Part model, mm, in its own coordinate system. Round coordinates to 2 decimals unless told otherwise and drop trailing zeros. Loops run counter-clockwise (first coordinate to the right, second up) from the corner with the lowest first, then second, coordinate; pieces in that order, holes last. Notation, with made-up numbers: (7, 18.5) - (40, 18.5) arc R29 ccw to (40, 53.5) - close; hole circle Ø8 at (47, -4). An arc over 180 degrees is marked (long way). Put each result on its own line as item: value.
Autodesk Inventor part; units mm, degrees
ref_plane "YZ Plane" through (0, 0, 0) normal (1, 0, 0) x (0, 1, 0)
ref_plane "XZ Plane" through (0, 0, 0) normal (0, 1, 0) x (-1, 0, 0)
ref_plane "XY Plane" through (0, 0, 0) normal (0, 0, 1) x (1, 0, 0)
sketch "Sketch2" plane through (0, 0, 0) normal (0, 0, 1) x (1, 0, 0)
  line L0 (307.5, 20) -> (347.5, 20)
  line L1 (347.5, 20) -> (347.5, -20)
  line L2 (347.5, -20) -> (307.5, -20)
  line L3 (307.5, -20) -> (307.5, 20)
  line L4 (307.5, 20) -> (347.5, -20) construction
  line L5 (347.5, 20) -> (307.5, -20) construction
  line L6 (327.5, 0) -> (-327.5, 0) construction
  line L7 (0, -327.5) -> (0, 327.5) construction
  line L8 (327.5, 0) -> (268.3955, 0) construction
  line L9 (327.5, 4.25) -> (268.3955, 4.25)
  line L10 (268.3955, -4.25) -> (327.5, -4.25)
  arc A0 (327.5, -4.25) -> (327.5, 4.25) centre (327.5, 0) ccw
  arc A1 (268.3955, 4.25) -> (268.3955, -4.25) centre (268.3955, 0) ccw
  line L11 (207.0955, 15.5) -> (297.2, 15.5) construction
  line L12 (207.0955, 13.9) -> (297.2, 13.9)
  line L13 (297.2, 17.1) -> (207.0955, 17.1)
  arc A2 (207.0955, 17.1) -> (207.0955, 13.9) centre (207.0955, 15.5) ccw
  arc A3 (297.2, 13.9) -> (297.2, 17.1) centre (297.2, 15.5) ccw
  line L14 (207.0955, -15.5) -> (297.2, -15.5) construction
  line L15 (207.0955, -17.1) -> (297.2, -17.1)
  line L16 (297.2, -13.9) -> (207.0955, -13.9)
  arc A4 (207.0955, -13.9) -> (207.0955, -17.1) centre (207.0955, -15.5) ccw
  arc A5 (297.2, -17.1) -> (297.2, -13.9) centre (297.2, -15.5) ccw
  arc A6 (-4.25, 268.3955) -> (4.25, 268.3955) centre (0, 268.3955) ccw
  line L17 (-13.9, 207.0955) -> (-13.9, 297.2)
  line L18 (-15.5, 207.0955) -> (-15.5, 297.2) construction
  line L19 (-17.1, 297.2) -> (-17.1, 207.0955)
  line L20 (17.1, 207.0955) -> (17.1, 297.2)
  line L21 (13.9, 297.2) -> (13.9, 207.0955)
  arc A7 (17.1, 297.2) -> (13.9, 297.2) centre (15.5, 297.2) ccw
  line L22 (20, 307.5) -> (-20, 307.5)
  line L23 (15.5, 207.0955) -> (15.5, 297.2) construction
  arc A8 (-17.1, 207.0955) -> (-13.9, 207.0955) centre (-15.5, 207.0955) ccw
  arc A9 (13.9, 207.0955) -> (17.1, 207.0955) centre (15.5, 207.0955) ccw
  line L24 (-20, 307.5) -> (-20, 347.5)
  line L25 (-20, 347.5) -> (20, 347.5)
  line L26 (20, 347.5) -> (20, 307.5)
  line L27 (-20, 307.5) -> (20, 347.5) construction
  line L28 (-20, 347.5) -> (20, 307.5) construction
  arc A10 (-13.9, 297.2) -> (-17.1, 297.2) centre (-15.5, 297.2) ccw
  line L29 (0, 327.5) -> (0, 268.3955) construction
  line L30 (4.25, 268.3955) -> (4.25, 327.5)
  arc A11 (4.25, 327.5) -> (-4.25, 327.5) centre (0, 327.5) ccw
  line L31 (-4.25, 327.5) -> (-4.25, 268.3955)
  arc A12 (-268.3955, -4.25) -> (-268.3955, 4.25) centre (-268.3955, 0) ccw
  line L32 (-207.0955, -13.9) -> (-297.2, -13.9)
  line L33 (-207.0955, -15.5) -> (-297.2, -15.5) construction
  line L34 (-297.2, -17.1) -> (-207.0955, -17.1)
  line L35 (-207.0955, 17.1) -> (-297.2, 17.1)
  line L36 (-297.2, 13.9) -> (-207.0955, 13.9)
  arc A13 (-297.2, 17.1) -> (-297.2, 13.9) centre (-297.2, 15.5) ccw
  line L37 (-307.5, 20) -> (-307.5, -20)
  line L38 (-207.0955, 15.5) -> (-297.2, 15.5) construction
  arc A14 (-207.0955, -17.1) -> (-207.0955, -13.9) centre (-207.0955, -15.5) ccw
  arc A15 (-207.0955, 13.9) -> (-207.0955, 17.1) centre (-207.0955, 15.5) ccw
  line L39 (-307.5, -20) -> (-347.5, -20)
  line L40 (-347.5, -20) -> (-347.5, 20)
  line L41 (-347.5, 20) -> (-307.5, 20)
  line L42 (-307.5, -20) -> (-347.5, 20) construction
  line L43 (-347.5, -20) -> (-307.5, 20) construction
  arc A16 (-297.2, -13.9) -> (-297.2, -17.1) centre (-297.2, -15.5) ccw
  line L44 (-327.5, 0) -> (-268.3955, 0) construction
  line L45 (-268.3955, 4.25) -> (-327.5, 4.25)
  arc A17 (-327.5, 4.25) -> (-327.5, -4.25) centre (-327.5, 0) ccw
  line L46 (-327.5, -4.25) -> (-268.3955, -4.25)
  arc A18 (4.25, -268.3955) -> (-4.25, -268.3955) centre (0, -268.3955) ccw
  line L47 (13.9, -207.0955) -> (13.9, -297.2)
  line L48 (15.5, -207.0955) -> (15.5, -297.2) construction
  line L49 (17.1, -297.2) -> (17.1, -207.0955)
  line L50 (-17.1, -207.0955) -> (-17.1, -297.2)
  line L51 (-13.9, -297.2) -> (-13.9, -207.0955)
  arc A19 (-17.1, -297.2) -> (-13.9, -297.2) centre (-15.5, -297.2) ccw
  line L52 (-20, -307.5) -> (20, -307.5)
  line L53 (-15.5, -207.0955) -> (-15.5, -297.2) construction
  arc A20 (17.1, -207.0955) -> (13.9, -207.0955) centre (15.5, -207.0955) ccw
  arc A21 (-13.9, -207.0955) -> (-17.1, -207.0955) centre (-15.5, -207.0955) ccw
  line L54 (20, -307.5) -> (20, -347.5)
  line L55 (20, -347.5) -> (-20, -347.5)
  line L56 (-20, -347.5) -> (-20, -307.5)
  line L57 (20, -307.5) -> (-20, -347.5) construction
  line L58 (20, -347.5) -> (-20, -307.5) construction
  arc A22 (13.9, -297.2) -> (17.1, -297.2) centre (15.5, -297.2) ccw
  line L59 (0, -327.5) -> (0, -268.3955) construction
  line L60 (-4.25, -268.3955) -> (-4.25, -327.5)
  arc A23 (-4.25, -327.5) -> (4.25, -327.5) centre (0, -327.5) ccw
  line L61 (4.25, -327.5) -> (4.25, -268.3955)
  line L62 (-307.5, 20) -> (-20, 307.5)
  line L63 (20, 307.5) -> (307.5, 20)
  line L64 (307.5, -20) -> (20, -307.5)
  line L65 (-20, -307.5) -> (-307.5, -20)
  point P0 (0, 0)
  point P1 (297.9478, 0)
  point P2 (252.1478, 15.5)
  point P3 (252.1478, -15.5)
  point P4 (15.5, 252.1478)
  point P5 (-15.5, 252.1478)
  point P6 (0, 297.9478)
  point P7 (-252.1478, 15.5)
  point P8 (-252.1478, -15.5)
  point P9 (-297.9478, 0)
  point P10 (-15.5, -252.1478)
  point P11 (15.5, -252.1478)
  point P12 (0, -297.9478)
  dimension "d148" = 40
  dimension "d149" = 655
  dimension "d154" = 59.1045
  dimension "d155" = 8.5
  dimension "d156" = 90.1045
  dimension "d157" = 3.2
  dimension "d171" = 31
  dimension "d172" = 10.3
  dimension "d173" = 10.3
  dimension "d176" = 360
extrude "Extrusion10" add sketch "Sketch2" against normal blind 10 contours L0 L1 L2 L3 L10 A0 L9 | L3 L9 A1 L10 L64 L52 L61 A18 L60 L65 L37 L46 A12 L45 L62 L22 L31 A6 L30 L63 | L22 L30 A11 L31 L24 L25 L26 | L54 L55 L56 L52 L60 A23 L61 | L37 L45 A17 L46 L39 L40 L41
fillet "Fillet8" radius 4 16 edges at (20, 347.5, -5) (-20, 347.5, -5) (-20, 307.5, -5) (-307.5, 20, -5) (-347.5, 20, -5) (-347.5, -20, -5) (347.5, 20, -5) (-20, -307.5, -5) (-20, -347.5, -5) (20, 307.5, -5) (20, -347.5, -5) (347.5, -20, -5) (307.5, -20, -5) (20, -307.5, -5) (307.5, 20, -5) (-307.5, -20, -5)
equation "\"ring_inner_diam\" = 565"
equation "\"ring_outer_diam\" = 615"
equation "\"dist_motor_bar\" = 10.3"
equation "\"motor_slot_diam\" = 3.2"
equation "\"motor_slot_length\" = 90.1045"
equation "\"bar_slot_diam\" = 8.5"
equation "\"bar_slot_length\" = 59.1045"
equation "\"diag_dist_bar_holes_old_fridge\" = 536.791"
equation "\"motor_dist_slots\" = 31"
properties part number "base_plate" material "Aluminum 6061"
1. Band-saw the part on B-B (z = -5.25). Give the number of separate pieces and of enclosed holes in the cut face, plus the area to 3 significant figures.
A:
separate pieces: 1
enclosed holes: 12
area: 215,000 mm²
2. Band-saw the part on C-C (y = -165.5). List the corners of the cut face in (x, z).
A:
outline: (-162, -10) - (162, -10) - (162, 0) - (-162, 0) - close
3. Band-saw the part on D-D (x = 46.5). List the corners of the cut face in (y, z).
A:
outline: (-281, -10) - (281, -10) - (281, 0) - (-281, 0) - close
4. Probe line 1 along Y through (x, z) = (1, -3); line 2 along X through (y, z) = (-235.5, -3); line 3 along Y through (x, z) = (295.5, -3.75). List the from-to ranges inside material, lowest first. Write a range as [from, to].
A:
line 1: y = [-347.5, -331.63], [-264.26, 264.26], [331.63, 347.5]
line 2: x = [-92, -17.1], [-13.9, 13.9], [17.1, 92]
line 3: y = [-32, -17.1], [-13.9, -4.25], [4.25, 13.9], [17.1, 32]
5. Pin check, flat tips, straight feed: P1, Ø3, axis at y = 295.5, z = -5.5, coming from the -X side; P2, Ø3, axis at y = -312, z = -5, coming from the +X side; P3, Ø5, axis at x = 325.5, z = -3, coming from the -Y side. Stop position of each tip, or through.
A:
P1: stops at x = -33.5
P2: stops at x = 20
P3: stops at y = -20
6. Band-saw the part on A-A (x = -287.5). List the corners of the cut face in (y, z), plus the area to 3 significant figures.
A:
outline: (-40, -10) - (-17.1, -10) - (-17.1, 0) - (-40, 0) - close; (-13.9, -10) - (-4.25, -10) - (-4.25, 0) - (-13.9, 0) - close; (4.25, -10) - (13.9, -10) - (13.9, 0) - (4.25, 0) - close; (17.1, -10) - (40, -10) - (40, 0) - (17.1, 0) - close
area: 651 mm²
